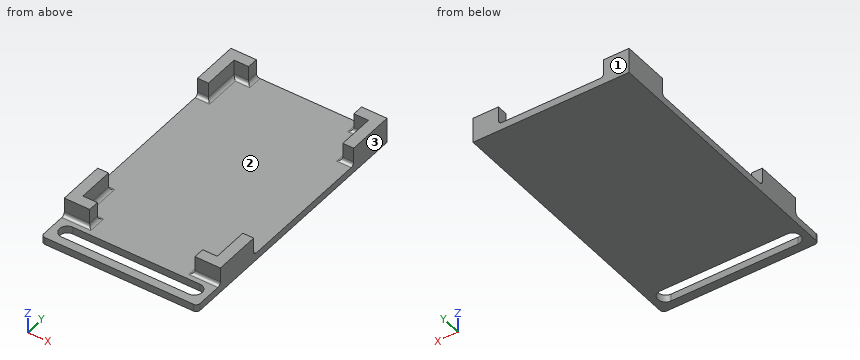
Autodesk Fusion 360 part; units mm, degrees
sketch "Sketch1" plane through (0, 0, 0) normal (0, 0, 1) x (1, 0, 0)
  line L0 (18.5, 29.5) -> (-18.5, 29.5) construction
  line L1 (-18.5, 29.5) -> (-18.5, -29.5) construction
  line L2 (-18.5, -29.5) -> (18.5, -29.5) construction
  line L3 (18.5, -29.5) -> (18.5, 29.5) construction
  line L4 (18.5, 29.5) -> (-18.5, -29.5) construction
  line L5 (-18.5, 29.5) -> (18.5, -29.5) construction
  line L6 (-18.5, 19.5) -> (-21.5, 19.5)
  line L7 (-21.5, 19.5) -> (-21.5, 32.5)
  line L8 (-21.5, 32.5) -> (-14.5, 32.5)
  line L9 (-14.5, 32.5) -> (-14.5, 29.5)
  line L10 (0, 29.5) -> (0, -29.5) construction
  line L11 (21.5, 32.5) -> (14.5, 32.5)
  line L12 (21.5, 19.5) -> (21.5, 32.5)
  line L13 (18.5, 19.5) -> (21.5, 19.5)
  line L14 (14.5, 32.5) -> (14.5, 29.5)
  line L15 (-18.5, 0) -> (18.5, 0) construction
  line L16 (-18.5, -19.5) -> (-21.5, -19.5)
  line L17 (-21.5, -19.5) -> (-21.5, -32.5)
  line L18 (-21.5, -32.5) -> (-14.5, -32.5)
  line L19 (-14.5, -32.5) -> (-14.5, -29.5)
  line L20 (21.5, -32.5) -> (14.5, -32.5)
  line L21 (14.5, -32.5) -> (14.5, -29.5)
  line L22 (21.5, -19.5) -> (21.5, -32.5)
  line L23 (18.5, -19.5) -> (21.5, -19.5)
  line L24 (14.5, 29.5) -> (18.5, 29.5)
  line L25 (18.5, 19.5) -> (18.5, 29.5)
  line L26 (-18.5, 29.5) -> (-18.5, 19.5)
  line L27 (-18.5, 29.5) -> (-14.5, 29.5)
  line L28 (-18.5, -19.5) -> (-18.5, -29.5)
  line L29 (-14.5, -29.5) -> (-18.5, -29.5)
  line L30 (14.5, -29.5) -> (18.5, -29.5)
  line L31 (18.5, -29.5) -> (18.5, -19.5)
  dimension "d1" = 59
  dimension "d2" = 37
  dimension "d3" = 13
  dimension "d4" = 3
  dimension "d5" = 4
  dimension "d6" = 3
extrude "Extrude1" add sketch "Sketch1" along normal blind 5 makes body 1 at (-21.5, 23.8333, 1.6667) makes body 2 at (-21.5, -23.8333, 1.6667) makes body 3 at (21.5, 23.8333, 1.6667) makes body 4 at (21.5, -23.8333, 1.6667)
sketch "Sketch2" plane through (0, 0, 0) normal (0, 0, -1) x (1, 0, 0)
  line L0 (-21.5, 19.5) -> (-18.5, 19.5)
  line L1 (-18.5, 19.5) -> (-18.5, 29.5)
  line L2 (-18.5, 29.5) -> (-14.5, 29.5)
  line L3 (-14.5, 29.5) -> (-14.5, 32.5)
  line L4 (-14.5, 32.5) -> (-21.5, 32.5)
  line L5 (-21.5, 32.5) -> (-21.5, 19.5)
  line L6 (-21.5, 32.5) -> (21.5, 32.5) construction
  line L7 (21.5, 32.5) -> (21.5, -32.5)
  line L8 (21.5, -32.5) -> (-21.5, -32.5)
  line L9 (-21.5, -32.5) -> (-21.5, 32.5)
  line L10 (5, 32.5) -> (-5, 32.5) construction
  line L11 (0, -32.5) -> (0, 32.5) construction
  line L12 (21.5, 32.5) -> (-21.5, 32.5)
  line L13 (-21.5, 32.5) -> (-21.5, 41.5)
  line L14 (-21.5, 41.5) -> (21.5, 41.5)
  line L15 (21.5, 41.5) -> (21.5, 32.5)
  line L16 (21.5, 37) -> (-21.5, 37) construction
  line L17 (0, 32.5) -> (0, 41.5) construction
  line L18 (17.5, 39.15) -> (-17.5, 39.15)
  arc A0 (-17.5, 39.15) -> (-17.5, 34.85) centre (-17.5, 37) ccw
  line L19 (-17.5, 34.85) -> (17.5, 34.85)
  arc A1 (17.5, 34.85) -> (17.5, 39.15) centre (17.5, 37) ccw
  line L20 (17.5, 37) -> (-17.5, 37) construction
  point P0 (0, 37)
  dimension "d9" = 10
  dimension "d10" = 9
  dimension "d11" = 35
  dimension "d12" = 4.3
extrude "Extrude2" add sketch "Sketch2" along normal blind 2 bodies 1 2 3 4
fillet "Fillet1" radius 1 16 edges at (-20, 19.5, 0) (-18.5, 24.5, 0) (-16.5, 29.5, 0) (-14.5, 31, 0) (14.5, 31, 0) (16.5, 29.5, 0) (18.5, 24.5, 0) (20, 19.5, 0) (20, -19.5, 0) (18.5, -24.5, 0) (16.5, -29.5, 0) (14.5, -31, 0) (-14.5, -31, 0) (-16.5, -29.5, 0) (-18.5, -24.5, 0) (-20, -19.5, 0) on bodies 1
fillet "Fillet1" radius 1 4 edges at (-21.5, -41.5, -1) (21.5, -41.5, -1) (18, -32.5, 0) (-18, -32.5, 0) on bodies 1
The listing builds one solid part. Answer for the finished solid, in the listing's coordinates (mm). Face numbers are marked on the shaded views. Give positions to 0.01 mm unless a question says otherwise; leave off trailing zeros. Write each loop counter-clockwise with the first axis right and the second up, starting at its lowest first coordinate (ties: lowest second). Pieces come first, ordered by that corner, then holes.
1) Section D-D (z = 2.5) is taken. Write down the section's boundary in (x, y), and give its area (3 significant figures).
2) For a pull along Y with two mould halves and no side action, classify the marked faces 1, 2 and 3 as pulls with the +Y half, pulls with the -Y half, needs draft (parallel to the pull), parting line crosses it, or undercut.
3) Given P1, Ø3, axis at x = 19.5, z = 2, coming from the -Y side; P2, Ø0.9, axis at x = 20.5, z = 4, coming from the -Y side; P3, Ø4, axis at x = -5.5, y = 17.5, coming from the +Z side, each flat-ended and moving along its own axis, determine where each tip first touches the part or whether it passes through.
4) Section B-B (x = -16.5) is taken. Write down the section's boundary in (y, z), and give its area (3 significant figures).
5) Find the intervals of material crossed by L1, parallel to Y at x = -6, z = -0.5; L2, parallel to Y at x = -19, z = 4; L3, parallel to X at y = 22, z = 4, in increasing order.
6) Section C-C (z = -0.75) is taken. Write down the section's boundary in (x, y).
7) Section A-A (y = -37) is taken. Write down the section's boundary in (x, z), and give its area (3 significant figures).
Response:
1. outline: (-21.5, -32.5) - (-14.5, -32.5) - (-14.5, -29.5) - (-18.5, -29.5) - (-18.5, -19.5) - (-21.5, -19.5) - close; (-21.5, 19.5) - (-18.5, 19.5) - (-18.5, 29.5) - (-14.5, 29.5) - (-14.5, 32.5) - (-21.5, 32.5) - close; (14.5, -32.5) - (21.5, -32.5) - (21.5, -19.5) - (18.5, -19.5) - (18.5, -29.5) - (14.5, -29.5) - close; (14.5, 29.5) - (18.5, 29.5) - (18.5, 19.5) - (21.5, 19.5) - (21.5, 32.5) - (14.5, 32.5) - close
1. area: 204 mm2
2. face 1: pulls with the +Y half
2. face 2: undercut
2. face 3: needs draft
3. P1: stops at y = -32.63
3. P2: stops at y = -32.5
3. P3: stops at z = 0
4. outline: (-41.5, -2) - (-39.15, -2) - (-39.15, 0) - (-41.5, 0) - close; (-34.85, -2) - (32.5, -2) - (32.5, 5) - (29.5, 5) - (29.5, 1) arc R1 cw to (28.5, 0) - (-28.5, 0) arc R1 cw to (-29.5, 1) - (-29.5, 5) - (-32.5, 5) - (-32.5, 1) arc R1 cw to (-33.5, 0) - (-34.85, 0) - close
4. area: 170 mm2
5. L1: y = -41.5 to -39.15, -34.85 to 32.5
5. L2: y = -32.5 to -19.5, 19.5 to 32.5
5. L3: x = -21.5 to -18.5, 18.5 to 21.5
6. outline: (-21.5, -40.5) arc R1 ccw to (-20.5, -41.5) - (20.5, -41.5) arc R1 ccw to (21.5, -40.5) - (21.5, 32.5) - (-21.5, 32.5) - close; hole (-17.5, -39.15) - (17.5, -39.15) arc R2.15 ccw to (17.5, -34.85) - (-17.5, -34.85) arc R2.15 ccw to start
7. outline: (-21.5, -2) - (-19.65, -2) - (-19.65, 0) - (-21.5, 0) - close; (19.65, -2) - (21.5, -2) - (21.5, 0) - (19.65, 0) - close
7. area: 7.40 mm2
